```python
from build123d import *

# Parameters (mm, degrees)
CYLINDER_R           = 20
CYLINDER_DEPTH       = 45
POCKET_DEPTH         = 164.569323
POCKET_DEPTH_BACK    = 164.569323
POCKET001_DEPTH      = 164.569324
POCKET001_DEPTH_BACK = 164.569324
SKETCH002_R          = 5
POCKET002_DEPTH      = 20.001
POCKET002_DEPTH_BACK = 20.001


with BuildPart() as part:
    # Cylinder → Cylinder (join)
    with BuildSketch(Plane.XY):
        Circle(CYLINDER_R)
    extrude(amount=CYLINDER_DEPTH)

    # Sketch → Pocket (cut, two sides)
    with BuildSketch(Plane.XZ) as pocket_sk:
        with BuildLine():
            ThreePointArc((-10, 10), (-7.071068, 2.928932), (0, 0))
            Line((-30, 0), (0, 0))
            Line((-30, 40), (-30, 0))
            Line((-20, 40), (-30, 40))
            ThreePointArc((-10, 30), (-12.928932, 37.071068), (-20, 40))
            Line((-10, 10), (-10, 30))
        make_face()
    pocket = extrude(amount=-POCKET_DEPTH, mode=Mode.SUBTRACT) + extrude(pocket_sk.sketch, amount=POCKET_DEPTH_BACK, mode=Mode.SUBTRACT)

    # Mirrored: Pocket across Sketch V_Axis
    add(pocket.mirror(Plane(origin=(0, 0, 0), x_dir=(0, -1, 0), z_dir=(1, 0, 0))), mode=Mode.SUBTRACT)

    # Sketch001 → Pocket001 (cut, two sides)
    with BuildSketch(Plane.YZ) as pocket001_sk:
        with BuildLine():
            Line((-12, 0), (-12, 29))
            ThreePointArc((-6, 35), (-10.242641, 33.242641), (-12, 29))
            Line((-6, 35), (0, 35))
            Line((0, 35), (0, 0))
            Line((0, 0), (-12, 0))
        make_face()
    pocket001 = extrude(amount=-POCKET001_DEPTH, mode=Mode.SUBTRACT) + extrude(pocket001_sk.sketch, amount=POCKET001_DEPTH_BACK, mode=Mode.SUBTRACT)

    # Mirrored001: Pocket001 across Sketch001 V_Axis
    add(pocket001.mirror(Plane(origin=(0, 0, 0), x_dir=(1, 0, 0), z_dir=(0, 1, 0))), mode=Mode.SUBTRACT)

    # Sketch002 → Pocket002 (cut, two sides)
    with BuildSketch(Plane.XZ) as pocket002_sk:
        with Locations((0, 12)):
            Circle(SKETCH002_R)
    extrude(amount=-POCKET002_DEPTH, mode=Mode.SUBTRACT)
    extrude(pocket002_sk.sketch, amount=POCKET002_DEPTH_BACK, mode=Mode.SUBTRACT)


solid = part.part
```
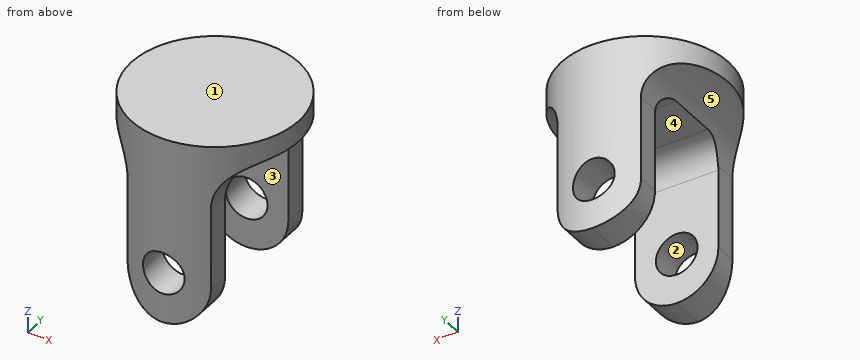
Input: part model. Units: mm. Frame: model coordinates. Face numbers are marked on the shaded views. A direction names the side the tool comes from. Give positions to 0.01 mm unless a question says otherwise; leave off trailing zeros. Write each loop counter-clockwise with the first axis right and the second up, starting at its lowest first coordinate (ties: lowest second). Pieces come first, ordered by that corner, then holes. Notation, with made-up numbers: (58.5, 22.5) - (107.5, 22.5) arc R14 cw to (107.5, 43.5) - close; hole circle Ø9 at (16.5, 56.5). An arc over 180 degrees is marked (long way). Write item = value, one per line. Start each with the question number.
1. Section query C-C, the plane z = 14. Output: boundary loops of the cut face in (x, y).
2. Ray query, L1, parallel to Z at x = 0, y = -17; L2, parallel to X at y = 14.5, z = 12; L3, parallel to X at y = 18.25, z = 12. Return the intervals inside material, ascending.
3. Section query A-A, the plane z = 25. Output: boundary loops of the cut face in (x, y).
4. Section query D-D, the plane y = -14. Output: boundary loops of the cut face in (x, z).
5. First-contact query: pin 1 Ø1.6 at (y, z) = (14, 15.5) entering from +X; pin 2 Ø1 at (x, z) = (-10, 38.5) entering from -Y; pin 3 Ø6 at (y, z) = (15.5, 16.5) entering from -X. Flat tips, straight axial feed; report the tip coordinate or a pass-through.
6. Mould query, pull axis Z, two halves, no side actions, for the marked faces 1, 2 and 3. Classes: released by +Z, released by -Z, zero draft, split by the parting line, or undercut.
7. Section query B-B, the plane x = -1.5. Output: boundary loops of the cut face in (y, z), then the cut area to 3 significant figures.
8. Access query for the marked faces 4 and 5. Directions: +Z, -Z, +X, -X, +Y, -Y. A direction counts if a zero-diameter tool reaches every point of the face in a straight line with its end or side. Return the directions, or none.
Check sheet entries:
q1.outline = (-10, -17.32) arc R20 ccw to (-4.58, -19.47) - (-4.58, -12) - (-10, -12) - close; (-10, 12) - (-4.58, 12) - (-4.58, 19.47) arc R20 ccw to (-10, 17.32) - close; (4.58, -19.47) arc R20 ccw to (10, -17.32) - (10, -12) - (4.58, -12) - close; (4.58, 12) - (10, 12) - (10, 17.32) arc R20 ccw to (4.58, 19.47) - close
q2.L1 = 0 to 7, 17 to 45
q2.L2 = -10 to -5, 5 to 10
q2.L3 = -8.18 to -5, 5 to 8.18
q3.outline = (-10, -17.32) arc R20 ccw to (10, -17.32) - (10, -12) - (-10, -12) - close; (-10, 12) - (10, 12) - (10, 17.32) arc R20 ccw to (-10, 17.32) - close
q4.outline = (-14.28, 38.2) arc R10 cw to (-10, 30) - (-10, 10) arc R10 ccw to (0, 0) arc R10 ccw to (10, 10) - (10, 30) arc R10 cw to (14.28, 38.2) - (14.28, 45) - (-14.28, 45) - close; hole circle Ø10 at (0, 12)
q5.pin_1 = 10
q5.pin_2 = -17.6
q5.pin_3 = -10
q6.face_1 = released by +Z
q6.face_2 = undercut
q6.face_3 = zero draft
q7.outline = (-19.94, 0.11) - (-12, 0.11) - (-12, 7.23) - (-19.94, 7.23) - close; (-19.94, 16.77) - (-12, 16.77) - (-12, 29) arc R6 cw to (-6, 35) - (6, 35) arc R6 cw to (12, 29) - (12, 16.77) - (19.94, 16.77) - (19.94, 45) - (-19.94, 45) - close; (12, 0.11) - (19.94, 0.11) - (19.94, 7.23) - (12, 7.23) - close
q7.area = 817 mm2
q8.face_4 = -Z, +X, -X
q8.face_5 = -Z, -X, +Y, -Y
